```python
from build123d import *

# Parameters (mm, degrees)
F1_DEPTH = 203.2
F2_W     = 25.4
F2_H     = 101.6
F3_DEPTH = 25.4
F4_W     = 50.8
F4_H     = 101.6
F5_DEPTH = 25.4
F7_DEPTH = 50.8
F8_W     = 101.6
F8_H     = 50.8
F9_DEPTH = 25.4


with BuildPart() as f1:
    # F0 (on Right) → F1 (new body)
    with BuildSketch(Plane.YZ):
        Polygon((12.87863, -0.538062), (-37.92137, -0.538062), (-37.92137, -25.938062), (63.67863, -25.938062), (63.67863, -0.538062), (63.67863, 75.661938), (12.87863, 75.661938), align=None)
    extrude(amount=F1_DEPTH)

    # F2 (on face) → F3 (cut)
    with BuildSketch(Plane.XY.offset(-0.538062)):
        with Locations((-25.22137, -101.6)):
            Rectangle(F2_W, F2_H)
    extrude(amount=-F3_DEPTH, mode=Mode.SUBTRACT)

    # F4 (on face) → F5 (cut)
    with BuildSketch(Plane.XY.offset(75.661938)):
        with Locations((38.27863, -101.6)):
            Rectangle(F4_W, F4_H)
    extrude(amount=-F5_DEPTH, mode=Mode.SUBTRACT)

    # F6 (on face) → F7 (cut)
    with BuildSketch(Plane.XZ.offset(-12.87863)):
        Polygon((203.2, 75.661938), (177.8, 75.661938), (203.2, 50.261938), align=None)
        Polygon((0, 50.261938), (25.4, 75.661938), (0, 75.661938), align=None)
    extrude(amount=-F7_DEPTH, mode=Mode.SUBTRACT)

    # F8 (on face) → F9 (cut)
    with BuildSketch(Plane.XY.offset(75.661938)):
        with Locations((101.6, 38.27863)):
            Rectangle(F8_W, F8_H)
    extrude(amount=-F9_DEPTH, mode=Mode.SUBTRACT)


solid = f1.part
```
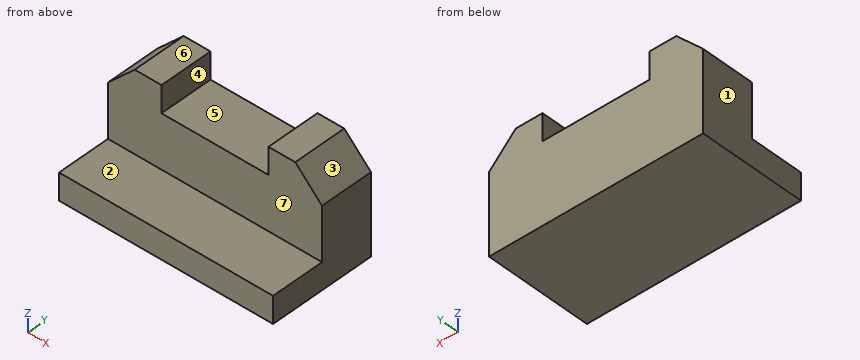
Here's how the part is built. I have some questions about the finished solid (model axes, mm). Face numbers are marked on the shaded views. A direction names the side the tool comes from. Give positions to 0.01 mm unless a question says otherwise; leave off trailing zeros. Loops run counter-clockwise (first coordinate to the right, second up) from the corner with the lowest first, then second, coordinate; pieces in that order, holes last. Notation, with made-up numbers: M -22.5,-9 L 21.5,-9 A30 cw 21.5,13 Z; hole C -10.75,85.5 d3. An arc over 180 degrees is marked long. Use one line per item in the form item = value. Start each with the question number.
Q1. Thinking about a two-plate mould opening in X: for the marked faces 1, 2, 3 and 4, which applies, +X half, -X half, draft (parallel to the pull), parting line (faces both ways), or undercut?
Q2. Will these pins go through, and if not, where does the flat tip stop? pin 1 Ø23 at (x, z) = (101.5, 35.5) entering from -Y; pin 2 Ø8 at (y, z) = (-4.5, 0.5) entering from +X; pin 3 Ø12.5 at (y, z) = (45, 65) entering from -X; pin 4 Ø12 at (x, z) = (118, 57) entering from -Y.
Q3. If we section it at B-B (z = 64.5): Write out the boundary of the cut face in (x, y).
Q4. Which directions (+Z, -Z, +X, -X, +Y, -Y) give clear straight access to the entire face, cutting with the end or side of a thin tool? Please do the marked faces 5, 6 and 7.
Q5. I need wall thicknesses on line 1 along Z through (x, y) = (80, 40); line 2 along Z through (x, y) = (134, -30); line 3 along Y through (x, z) = (75.5, 25.5). Which ranges of each line are inside material? Lowest first, please.
Q6. If we section it at A-A (y = 15.5): Write out the boundary of the cut face in (x, z), then the cut area to 3 significant figures.
Q7. If we section it at D-D (z = 24.5): Write out the boundary of the cut face in (x, y).
Q8. If we section it at C-C (x = 46): Write out the boundary of the cut face in (y, z).
Taken from the geometry:
q1.face_1 = -X half
q1.face_2 = draft
q1.face_3 = +X half
q1.face_4 = undercut
q2.pin_1 = 12.88
q2.pin_2 = 203.2
q2.pin_3 = 8.49
q2.pin_4 = through
q3.outline = M 14.24,12.88 L 50.8,12.88 L 50.8,63.68 L 14.24,63.68 Z; M 152.4,12.88 L 188.96,12.88 L 188.96,63.68 L 152.4,63.68 Z
q4.face_5 = +Z, +Y, -Y
q4.face_6 = +Z, +X, -X, +Y, -Y
q4.face_7 = +Z, +X, -X, -Y
q5.line_1 = -25.94 to 50.26
q5.line_2 = -25.94 to -0.54
q5.line_3 = 12.88 to 63.68
q6.outline = M 0,-25.94 L 203.2,-25.94 L 203.2,50.26 L 177.8,75.66 L 152.4,75.66 L 152.4,50.26 L 50.8,50.26 L 50.8,75.66 L 25.4,75.66 L 0,50.26 Z
q6.area = 17,400 mm^2
q7.outline = M 0,12.88 L 203.2,12.88 L 203.2,63.68 L 0,63.68 Z
q8.outline = M -37.92,-25.94 L 63.68,-25.94 L 63.68,75.66 L 12.88,75.66 L 12.88,-0.54 L -37.92,-0.54 Z
